For this review, use the dimensioned drawing (mm, ordinates from the lowest corner) and the shaded views. Coordinates: 2 decimals unless noted, no trailing zeros. Loops run counter-clockwise (first coordinate to the right, second up) from the corner with the lowest first, then second, coordinate; pieces in that order, holes last. Notation, with made-up numbers: (26.25, 34.25) - (56.25, 34.25) arc R11 cw to (56.25, 44.25) - close; hole circle Ø7 at (85.5, -3). An arc over 180 degrees is marked (long way). Answer in a Markdown table with one row per item. Add a question column.
(1) Clearance check with flat-ended pins moving along their axes: pin 1 (1 mm diameter, centred on x = 39.5, z = 1.5, fed in from +Y); pin 2 (1.6 mm diameter, centred on y = 57.5, z = 2.5, fed in from +X) (3 decimals); pin 3 (1.6 mm diameter, centred on y = 53, z = 4, fed in from -X); pin 4 (1.5 mm diameter, centred on x = 23, z = 0.5, fed in from -Y). State where each tip first meets the part, or that it passes through.
(2) To check wall thickness, follow L1, parallel to X at y = 4, z = 4 (3 decimals); L2, parallel to X at y = 56, z = 2.7 (3 decimals); L3, parallel to Y at x = 50.8, z = 2.25. State the ranges of each line that lie inside material, in increasing order. Write a range as [from, to].
(3) We need section C-C, the plane z = 2.8. Write out the cut boundary in (x, y) (3 decimals), plus the area to 3 significant figures.
(4) We need section B-B, the plane y = 22.5. Write out the cut boundary in (x, z).
(5) We need section D-D, the plane y = 35. Write out the cut boundary in (x, z), plus the area to 3 significant figures.
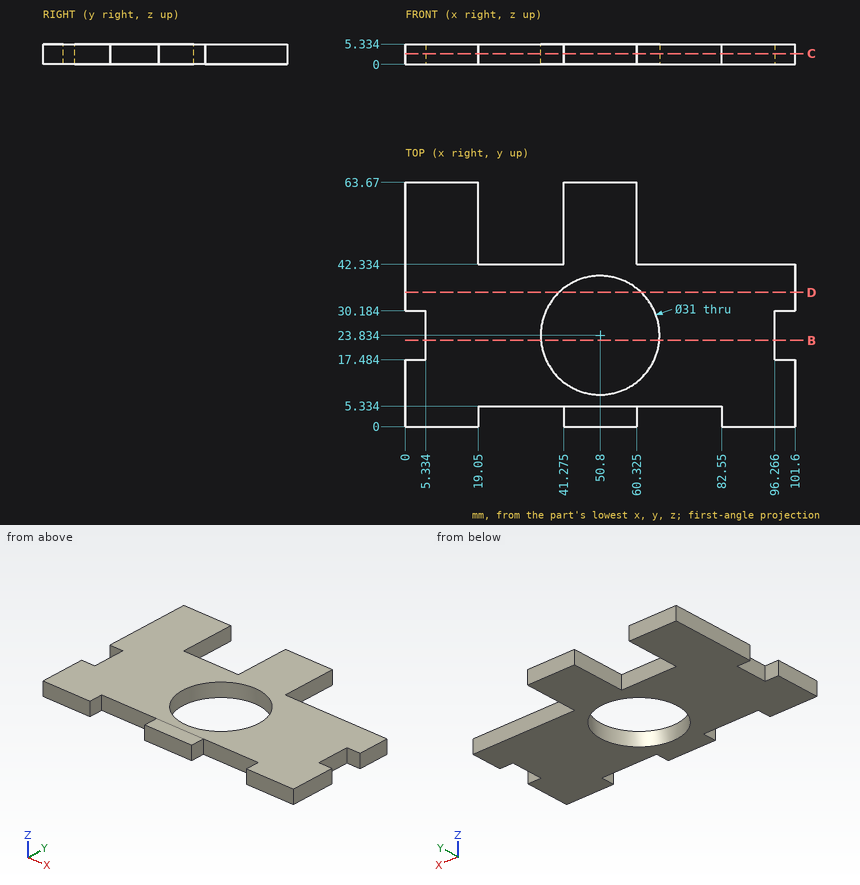
Responses:
| question | item | result |
|---|---|---|
| 1 | pin 1 | stops at y = 42.33 |
| 1 | pin 2 | stops at x = 60.325 |
| 1 | pin 3 | stops at x = 0 |
| 1 | pin 4 | stops at y = 5.33 |
| 2 | L1 | x = [0, 19.05], [41.275, 60.325], [82.55, 101.6] |
| 2 | L2 | x = [0, 19.05], [41.275, 60.325] |
| 2 | L3 | y = [0, 8.33], [39.33, 63.67] |
| 3 | outline | (0, 0) - (19.05, 0) - (19.05, 5.334) - (41.275, 5.334) - (41.275, 0) - (60.325, 0) - (60.325, 5.334) - (82.55, 5.334) - (82.55, 0) - (101.6, 0) - (101.6, 17.484) - (96.266, 17.484) - (96.266, 30.184) - (101.6, 30.184) - (101.6, 42.334) - (60.325, 42.334) - (60.325, 63.67) - (41.275, 63.67) - (41.275, 42.334) - (19.05, 42.334) - (19.05, 63.67) - (0, 63.67) - (0, 30.184) - (5.334, 30.184) - (5.334, 17.484) - (0, 17.484) - close; hole circle Ø31 at (50.8, 23.834) |
| 3 | area | 3,990 mm2 |
| 4 | outline | (5.33, 0) - (35.36, 0) - (35.36, 5.33) - (5.33, 5.33) - close; (66.24, 0) - (96.27, 0) - (96.27, 5.33) - (66.24, 5.33) - close |
| 5 | outline | (0, 0) - (40.05, 0) - (40.05, 5.33) - (0, 5.33) - close; (61.55, 0) - (101.6, 0) - (101.6, 5.33) - (61.55, 5.33) - close |
| 5 | area | 427 mm2 |
